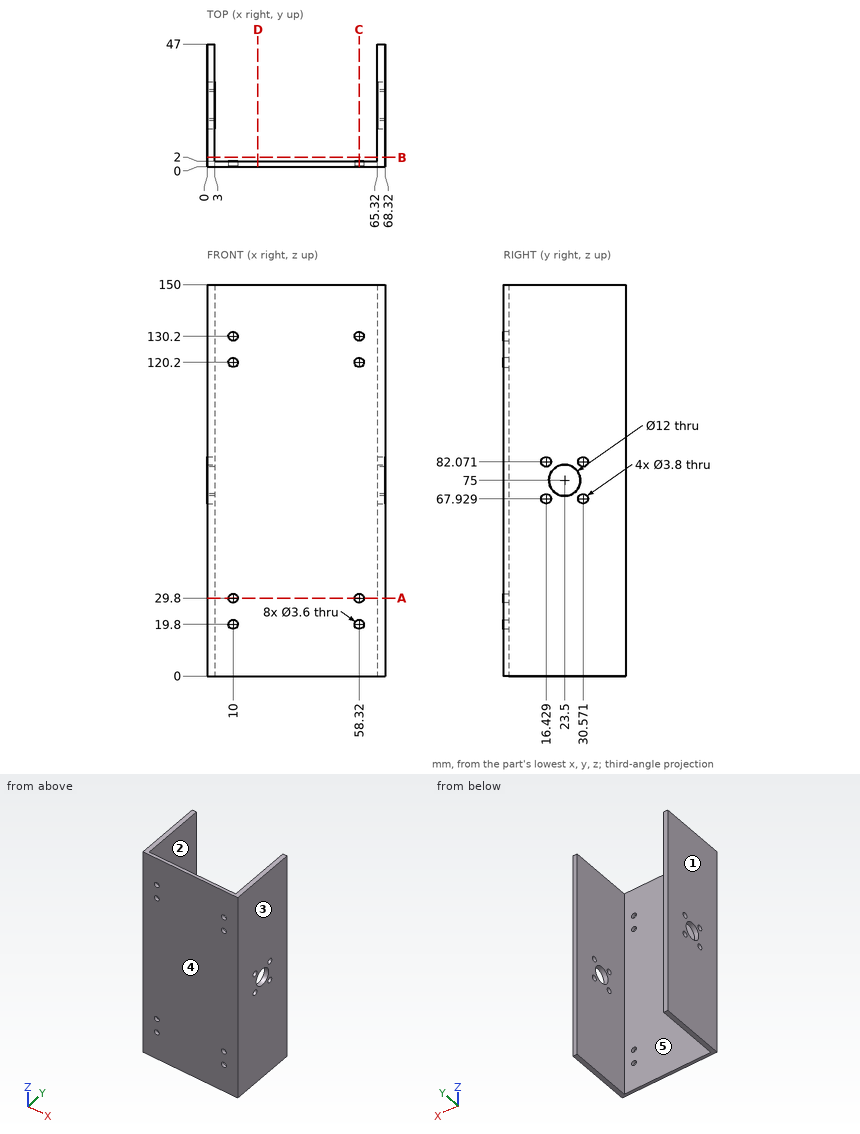
Drawing for the job (mm, zero at the part's lowest x, y, z). A direction names the side the tool comes from. Coordinates: 2 decimals unless noted, no trailing zeros. Order: outer loops, then holes, each group sorted by start corner. A loop starts at its lowest first (then second) coordinate and runs counter-clockwise, first axis right, second up.
Item 1: 3-axis set-ups, long thin cutter, end or side, ignore diameter. For the marked faces 1 and 2: which of +Z, -Z, +X, -X, +Y, -Y reach the whole face in a straight line?
Check sheet entries:
face 1: +Z, -Z, -X, +Y, -Y
face 2: +Z, -Z, +Y
Item 2: Band-saw the part on D-D on x = 19.5. List the corners of the cut face in (y, z), plus the area to 3 significant figures.
Check sheet entries:
outline: (0, 0) - (2, 0) - (2, 150) - (0, 150) - close
area: 300 mm2
Item 3: Band-saw the part on C-C on x = 58.32. List the corners of the cut face in (y, z).
Check sheet entries:
outline: (0, 0) - (2, 0) - (2, 18) - (0, 18) - close; (0, 21.6) - (2, 21.6) - (2, 28) - (0, 28) - close; (0, 31.6) - (2, 31.6) - (2, 118.4) - (0, 118.4) - close; (0, 122) - (2, 122) - (2, 128.4) - (0, 128.4) - close; (0, 132) - (2, 132) - (2, 150) - (0, 150) - close
Item 4: Band-saw the part on B-B on y = 3.5. List the corners of the cut face in (x, z), plus the area to 3 significant figures.
Check sheet entries:
outline: (0, 0) - (3, 0) - (3, 150) - (0, 150) - close; (65.32, 0) - (68.32, 0) - (68.32, 150) - (65.32, 150) - close
area: 900 mm2
Item 5: Drill centre lines: L1, parallel to Z at x = 58, y = 1; L2, parallel to X at y = 27, z = 49.5; L3, parallel to X at y = 1.1, z = 130.2. Where is each one in solid material? Low to high.
Check sheet entries:
L1: z = 0 to 18.03, 21.57 to 28.03, 31.57 to 118.43, 121.97 to 128.43, 131.97 to 150
L2: x = 0 to 3, 65.32 to 68.32
L3: x = 0 to 8.2, 11.8 to 56.52, 60.12 to 68.32
Item 6: Two-plate mould, pull along X, no slides. Class the marked faces 3, 4 and 5: +X half, -X half, draft (parallel to the pull), parting line (faces both ways), or undercut.
Check sheet entries:
face 3: +X half
face 4: draft
face 5: undercut
Item 7: Band-saw the part on A-A on z = 29.8. List the corners of the cut face in (x, y), plus the area to 3 significant figures.
Check sheet entries:
outline: (0, 0) - (8.2, 0) - (8.2, 2) - (3, 2) - (3, 47) - (0, 47) - close; (11.8, 0) - (56.52, 0) - (56.52, 2) - (11.8, 2) - close; (60.12, 0) - (68.32, 0) - (68.32, 47) - (65.32, 47) - (65.32, 2) - (60.12, 2) - close
area: 392 mm2
Item 8: Pin check, flat tips, straight feed: pin 1 Ø6 at (y, z) = (25, 53) entering from -X; pin 2 Ø4 at (x, z) = (58.32, 29.8) entering from +Y; pin 3 Ø2.5 at (y, z) = (16.43, 67.93) entering from -X. Stop position of each tip, or through.
Check sheet entries:
pin 1: stops at x = 0
pin 2: stops at y = 2
pin 3: passes through
